```python
from build123d import *

# Parameters (mm, degrees)
EXTRUDE_1_DEPTH     = 8
CUT_EXTRUDE_START   = -1
SKETCH_2_W          = 2.75
SKETCH_2_H          = 4.75
SKETCH_2_W_2        = 1.625
SKETCH_2_H_2        = 1.5
CUT_EXTRUDE_1_DEPTH = 25.734218465
SKETCH_3_W          = 0.5
SKETCH_3_H          = 1.625
EXTRUDE_2_DEPTH     = 2
CHAMFER_1_SIZE      = 1
SKETCH_4_W          = 1.625
SKETCH_4_H          = 1.5
EXTRUDE_3_DEPTH     = 1
CHAMFER_2_SIZE      = 3
SKETCH_5_W          = 5
SKETCH_5_H          = 1.925
EXTRUDE_4_DEPTH     = 16
SKETCH_6_W          = 6.5
SKETCH_6_H          = 1.925
SKETCH_6_W_2        = 28
EXTRUDE_5_DEPTH     = 5
SKETCH_7_R          = 1.75
CUT_EXTRUDE_2_DEPTH = 28.572631358


with BuildPart() as part:
    # Эскиз1 → Бобышка-Вытянуть1 (new body)
    with BuildSketch(Plane.XY):
        Polygon((-18.5, -6), (-12.5, -6), (-12.5, 6), (12.5, 6), (12.5, -6), (18.5, -6), (18.5, 10), (-18.5, 10), align=None)
    extrude(amount=EXTRUDE_1_DEPTH)

    # Эскиз2 → Вырез-Вытянуть1 (cut, through all)
    with BuildSketch(Plane.XZ.offset(6).offset(CUT_EXTRUDE_START)):
        with Locations((15.5, 4)):
            Rectangle(SKETCH_2_W, SKETCH_2_H)
        with Locations((13.3125, 4)):
            Rectangle(SKETCH_2_W_2, SKETCH_2_H_2)
        with Locations((-13.3125, 4)):
            Rectangle(SKETCH_2_W_2, SKETCH_2_H_2)
        Polygon((-14.125, 1.625), (-14.125, 3.25), (-14.125, 4.75), (-14.125, 6.375), (-16.875, 6.375), (-16.875, 1.625), align=None)
    extrude(amount=-CUT_EXTRUDE_1_DEPTH, mode=Mode.SUBTRACT)

    # Эскиз3 → Бобышка-Вытянуть2 (add)
    with BuildSketch(Plane(origin=(0, -5, 0), x_dir=(1, 0, 0), z_dir=(0, 1, 0))):
        with Locations((-14.375, -2.4375)):
            Rectangle(SKETCH_3_W, SKETCH_3_H)
        with Locations((-14.375, -5.5625)):
            Rectangle(SKETCH_3_W, SKETCH_3_H)
        with Locations((14.375, -5.5625)):
            Rectangle(SKETCH_3_W, SKETCH_3_H)
        with Locations((14.375, -2.4375)):
            Rectangle(SKETCH_3_W, SKETCH_3_H)
    extrude(amount=EXTRUDE_2_DEPTH)

    # Фаска1
    # the kernel refuses this chamfer: 1 mm, written as the material it adds along each edge
    with BuildSketch(Plane(origin=(-14.125, -3, 2.178317012), x_dir=(0.02749587661058563, 0.9996219169112968, 0), z_dir=(0, 0, 1))) as chamfer_1_piece_1_section:
        Polygon((CHAMFER_1_SIZE * 0.999621916911, CHAMFER_1_SIZE * 0.0274958766106), (-CHAMFER_1_SIZE * 0.0274958766106, CHAMFER_1_SIZE * 0.999621916911), (0, 0), align=None)
    chamfer_1_piece_1 = extrude(amount=6.768365976, mode=Mode.PRIVATE)
    chamfer_1_piece_1 = split(chamfer_1_piece_1, bisect_by=Plane(origin=(-14.625, -2.611111111, 2.714158506), z_dir=(1, 0, 0)), keep=Keep.TOP, mode=Mode.PRIVATE)
    chamfer_1_piece_1 = split(chamfer_1_piece_1, bisect_by=Plane(origin=(-14.347222222, -2.611111111, 3.25), z_dir=(0, 0, -1)), keep=Keep.TOP, mode=Mode.PRIVATE)
    add(chamfer_1_piece_1)
    with BuildSketch(Plane(origin=(-14.125, -3, 4.75), x_dir=(0.027495876610583895, 0.9996219169112968, 0), z_dir=(0, 0, 1))) as chamfer_1_piece_2_section:
        Polygon((CHAMFER_1_SIZE * 0.999621916911, CHAMFER_1_SIZE * 0.0274958766106), (-CHAMFER_1_SIZE * 0.0274958766106, CHAMFER_1_SIZE * 0.999621916911), (0, 0), align=None)
    chamfer_1_piece_2 = extrude(amount=1.625, mode=Mode.PRIVATE)
    chamfer_1_piece_2 = split(chamfer_1_piece_2, bisect_by=Plane(origin=(-14.625, -2.611111111, 5.5625), z_dir=(1, 0, 0)), keep=Keep.TOP, mode=Mode.PRIVATE)
    add(chamfer_1_piece_2)
    with BuildSketch(Plane(origin=(14.125, -3, 2.178317012), x_dir=(0.9996219169112968, -0.02749587661058651, -1.092729371642936e-15), z_dir=(0, 0, 1))) as chamfer_1_piece_3_section:
        Polygon((CHAMFER_1_SIZE * 0.999621916911, CHAMFER_1_SIZE * 0.0274958766106), (-CHAMFER_1_SIZE * 0.0274958766106, CHAMFER_1_SIZE * 0.999621916911), (0, 0), align=None)
    chamfer_1_piece_3 = extrude(amount=6.768365976, mode=Mode.PRIVATE)
    chamfer_1_piece_3 = split(chamfer_1_piece_3, bisect_by=Plane(origin=(14.347222222, -2.611111111, 3.25), z_dir=(0, 0, -1)), keep=Keep.TOP, mode=Mode.PRIVATE)
    chamfer_1_piece_3 = split(chamfer_1_piece_3, bisect_by=Plane(origin=(14.625, -2.611111111, 2.714158506), z_dir=(-1, 0, 0)), keep=Keep.TOP, mode=Mode.PRIVATE)
    add(chamfer_1_piece_3)
    with BuildSketch(Plane(origin=(14.125, -3, 4.75), x_dir=(0.9996219169112968, -0.02749587661058651, -1.092729371642936e-15), z_dir=(0, 0, 1))) as chamfer_1_piece_4_section:
        Polygon((CHAMFER_1_SIZE * 0.999621916911, CHAMFER_1_SIZE * 0.0274958766106), (-CHAMFER_1_SIZE * 0.0274958766106, CHAMFER_1_SIZE * 0.999621916911), (0, 0), align=None)
    chamfer_1_piece_4 = extrude(amount=1.625, mode=Mode.PRIVATE)
    chamfer_1_piece_4 = split(chamfer_1_piece_4, bisect_by=Plane(origin=(14.625, -2.611111111, 5.5625), z_dir=(-1, 0, 0)), keep=Keep.TOP, mode=Mode.PRIVATE)
    add(chamfer_1_piece_4)
    with BuildSketch(Plane(origin=(14.125, -3, 5.821682988), x_dir=(0.9996219169112968, -0.02749587661058651, 0), z_dir=(0, 0, -1))) as chamfer_1_piece_5_section:
        Polygon((CHAMFER_1_SIZE * 0.999621916911, -CHAMFER_1_SIZE * 0.0274958766106), (-CHAMFER_1_SIZE * 0.0274958766106, -CHAMFER_1_SIZE * 0.999621916911), (0, 0), align=None)
    chamfer_1_piece_5 = extrude(amount=6.768365976, mode=Mode.PRIVATE)
    chamfer_1_piece_5 = split(chamfer_1_piece_5, bisect_by=Plane(origin=(14.625, -2.611111111, 5.285841494), z_dir=(-1, 0, 0)), keep=Keep.TOP, mode=Mode.PRIVATE)
    chamfer_1_piece_5 = split(chamfer_1_piece_5, bisect_by=Plane(origin=(14.347222222, -2.611111111, 4.75), z_dir=(0, 0, 1)), keep=Keep.TOP, mode=Mode.PRIVATE)
    add(chamfer_1_piece_5)
    with BuildSketch(Plane(origin=(14.125, -3, 3.25), x_dir=(0.9996219169112968, -0.02749587661058651, 0), z_dir=(0, 0, -1))) as chamfer_1_piece_6_section:
        Polygon((CHAMFER_1_SIZE * 0.999621916911, -CHAMFER_1_SIZE * 0.0274958766106), (-CHAMFER_1_SIZE * 0.0274958766106, -CHAMFER_1_SIZE * 0.999621916911), (0, 0), align=None)
    chamfer_1_piece_6 = extrude(amount=4.196682988, mode=Mode.PRIVATE)
    chamfer_1_piece_6 = split(chamfer_1_piece_6, bisect_by=Plane(origin=(14.625, -2.611111111, 2.4375), z_dir=(-1, 0, 0)), keep=Keep.TOP, mode=Mode.PRIVATE)
    chamfer_1_piece_6 = split(chamfer_1_piece_6, bisect_by=Plane(origin=(14.347222222, -2.611111111, 0), z_dir=(0, 0, 1)), keep=Keep.TOP, mode=Mode.PRIVATE)
    add(chamfer_1_piece_6)
    with BuildSketch(Plane(origin=(-14.125, -3, 5.821682988), x_dir=(0.02749587661058563, 0.9996219169112968, 0), z_dir=(0, 0, -1))) as chamfer_1_piece_7_section:
        Polygon((CHAMFER_1_SIZE * 0.999621916911, -CHAMFER_1_SIZE * 0.0274958766106), (-CHAMFER_1_SIZE * 0.0274958766106, -CHAMFER_1_SIZE * 0.999621916911), (0, 0), align=None)
    chamfer_1_piece_7 = extrude(amount=6.768365976, mode=Mode.PRIVATE)
    chamfer_1_piece_7 = split(chamfer_1_piece_7, bisect_by=Plane(origin=(-14.347222222, -2.611111111, 4.75), z_dir=(0, 0, 1)), keep=Keep.TOP, mode=Mode.PRIVATE)
    chamfer_1_piece_7 = split(chamfer_1_piece_7, bisect_by=Plane(origin=(-14.625, -2.611111111, 5.285841494), z_dir=(1, 0, 0)), keep=Keep.TOP, mode=Mode.PRIVATE)
    add(chamfer_1_piece_7)
    with BuildSketch(Plane(origin=(-14.125, -3, 3.25), x_dir=(0.02749587661058563, 0.9996219169112968, 0), z_dir=(0, 0, -1))) as chamfer_1_piece_8_section:
        Polygon((CHAMFER_1_SIZE * 0.999621916911, -CHAMFER_1_SIZE * 0.0274958766106), (-CHAMFER_1_SIZE * 0.0274958766106, -CHAMFER_1_SIZE * 0.999621916911), (0, 0), align=None)
    chamfer_1_piece_8 = extrude(amount=4.196682988, mode=Mode.PRIVATE)
    chamfer_1_piece_8 = split(chamfer_1_piece_8, bisect_by=Plane(origin=(-14.625, -2.611111111, 2.4375), z_dir=(1, 0, 0)), keep=Keep.TOP, mode=Mode.PRIVATE)
    chamfer_1_piece_8 = split(chamfer_1_piece_8, bisect_by=Plane(origin=(-14.347222222, -2.611111111, 0), z_dir=(0, 0, 1)), keep=Keep.TOP, mode=Mode.PRIVATE)
    add(chamfer_1_piece_8)

    # Эскиз4 → Бобышка-Вытянуть3 (add)
    with BuildSketch(Plane(origin=(0, -5, 0), x_dir=(1, 0, 0), z_dir=(0, 1, 0))):
        with Locations((-13.3125, -4)):
            Rectangle(SKETCH_4_W, SKETCH_4_H)
        with Locations((13.3125, -4)):
            Rectangle(SKETCH_4_W, SKETCH_4_H)
    extrude(amount=EXTRUDE_3_DEPTH)

    # Фаска2
    chamfer_2_edges = [part.edges().sort_by_distance(p)[0] for p in [
        (12.5, 6, 6.375),
        (-12.5, 6, 6.375),
        (12.5, 6, 1.625),
        (-12.5, 6, 1.625),
    ]]
    chamfer(chamfer_2_edges, length=CHAMFER_2_SIZE)

    # Эскиз5 → Бобышка-Вытянуть4 (add, through all)
    with BuildSketch(Plane.XZ.offset(6)):
        with Locations((-21, 7.0375)):
            Rectangle(SKETCH_5_W, SKETCH_5_H)
        with Locations((-21, 0.9625)):
            Rectangle(SKETCH_5_W, SKETCH_5_H)
        with Locations((21, 7.0375)):
            Rectangle(SKETCH_5_W, SKETCH_5_H)
        with Locations((21, 0.9625)):
            Rectangle(SKETCH_5_W, SKETCH_5_H)
    extrude(amount=-EXTRUDE_4_DEPTH)

    # Эскиз6 → Бобышка-Вытянуть5 (add)
    with BuildSketch(Plane(origin=(0, 10, 0), x_dir=(1, 0, 0), z_dir=(0, 1, 0))):
        with Locations((-20.25, -0.9625)):
            Rectangle(SKETCH_6_W, SKETCH_6_H)
        with Locations((0, -0.9625)):
            Rectangle(SKETCH_6_W_2, SKETCH_6_H)
        with Locations((20.25, -0.9625)):
            Rectangle(SKETCH_6_W, SKETCH_6_H)
        Polygon((-16.875, -6.375), (-16.875, -6.075), (-23.5, -6.075), (-23.5, -8), (23.5, -8), (23.5, -6.075), (16.875, -6.075), (16.875, -6.375), (14.125, -6.375), (14.125, -6.075), (-14.125, -6.075), (-14.125, -6.375), align=None)
    extrude(amount=EXTRUDE_5_DEPTH)

    # Эскиз7 → Вырез-Вытянуть2 (cut, through all)
    with BuildSketch(Plane.XZ.offset(-6)):
        with Locations((-6.25, 4)):
            Circle(SKETCH_7_R)
        with Locations((6.25, 4)):
            Circle(SKETCH_7_R)
    extrude(amount=-CUT_EXTRUDE_2_DEPTH, mode=Mode.SUBTRACT)


solid = part.part
```
For this review, take the finished solid that the model builds, in its own axes (mm). A direction names the side the tool comes from. Round coordinates to 2 decimals unless told otherwise and drop trailing zeros. Loops run counter-clockwise (first coordinate to the right, second up) from the corner with the lowest first, then second, coordinate; pieces in that order, holes last.
Q1. Add section A-A on y = 12.25. Write out the cut boundary in (x, z) (3 decimals), plus the area to 3 significant figures.
Result sheet:
outline: (-23.5, 0) - (-17, 0) - (-17, 1.925) - (-23.5, 1.925) - close; (-23.5, 6.075) - (-16.875, 6.075) - (-16.875, 6.375) - (-14.125, 6.375) - (-14.125, 6.075) - (14.125, 6.075) - (14.125, 6.375) - (16.875, 6.375) - (16.875, 6.075) - (23.5, 6.075) - (23.5, 8) - (-23.5, 8) - close; (-14, 0) - (14, 0) - (14, 1.925) - (-14, 1.925) - close; (17, 0) - (23.5, 0) - (23.5, 1.925) - (17, 1.925) - close
area: 168 mm2
Q2. Add section C-C on z = 4. Write out the cut boundary in (x, y) (3 decimals), plus the area to 3 significant figures.
Result sheet:
outline: (-18.5, -6) - (-12.5, -6) - (-12.5, -4) - (-14.125, -4) - (-14.125, -5) - (-16.875, -5) - (-16.875, 10) - (-18.5, 10) - close; (-12.5, 6) - (-8, 6) - (-8, 10) - (-12.5, 10) - close; (-4.5, 6) - (4.5, 6) - (4.5, 10) - (-4.5, 10) - close; (8, 6) - (12.5, 6) - (12.5, 10) - (8, 10) - close; (12.5, -6) - (18.5, -6) - (18.5, 10) - (16.875, 10) - (16.875, -5) - (14.125, -5) - (14.125, -4) - (12.5, -4) - close
area: 136 mm2
Q3. Add section D-D on x = -16. Write out the cut boundary in (y, z) (3 decimals).
Result sheet:
outline: (-6, 0) - (10, 0) - (10, 1.625) - (-5, 1.625) - (-5, 6.375) - (15, 6.375) - (15, 8) - (-6, 8) - close
Q4. Add section B-B on x = -6.25. Write out the cut boundary in (y, z) (3 decimals).
Result sheet:
outline: (6, 0) - (15, 0) - (15, 1.925) - (10, 1.925) - (10, 2.25) - (6, 2.25) - close; (6, 5.75) - (10, 5.75) - (10, 6.075) - (15, 6.075) - (15, 8) - (6, 8) - close
Q5. Machinability: for faces 1 (the face through (-16, 2, 1.625)), 2 (the face through (13, 3, 4.75)), 3 (the face through (0, 12, 1.925)), 4 (the face through (11, 4.5, 1.6)), 5 (the face through (14, 12, 1)), which of the approach directions +Z, -Z, +X, -X, +Y, -Y give a long, thin tool a straight path to every point of the face, cutting with its end or side? Answer none if there is none.
Result sheet:
face 1: +Y
face 2: none
face 3: +X, -X, +Y
face 4: +Z, -Z, -Y
face 5: -Z, +Y
Q6. Mouldability with a two-part tool opening along X and no side actions: class faces 6 (the face through (0, 7, 0)), 7 (the face through (12.5, -1, 3)), 8 (the face through (23.5, 4, 1)) as +X half, -X half, draft (parallel to the pull), parting line (faces both ways), or undercut.
Result sheet:
face 6: draft
face 7: undercut
face 8: +X half
Q7. To check wall thickness, follow line 1 along X through (y, z) = (-3.25, 6.5); line 2 along Z through (x, y) = (8.5, 11.75) (3 decimals); line 3 along X through (y, z) = (-4, 5.5) (3 decimals). State the ranges of each line that lie inside material, in increasing order.
Result sheet:
line 1: x = -23.5 to -12.5, 12.5 to 23.5
line 2: z = 0 to 1.925, 6.075 to 8
line 3: x = -18.5 to -16.875, -14.625 to -12.5, 12.5 to 14.625, 16.875 to 18.5
Q8. Insertion check: pin 1 Ø0.8 at (y, z) = (3.5, 2.5) entering from -X; pin 2 Ø1.5 at (x, z) = (4.5, 4.5) entering from +Y; pin 3 Ø12 at (x, y) = (13, 7.5) entering from -Z; pin 4 Ø1 at (y, z) = (8.5, 5) entering from +X. Each pin has a flat end and moves straight along its axis. Give the tip position at first contact, or say it passes through.
Result sheet:
pin 1: stops at x = -18.5
pin 2: stops at y = 10
pin 3: stops at z = 0
pin 4: stops at x = 18.5
